```python
from build123d import *

# Parameters (mm, degrees)
F0_W     = 118.5
F0_H     = 123.5
F1_DEPTH = 1
F2_W     = 110
F2_H     = 115
F3_DEPTH = 25
F5_DEPTH = 1


with BuildPart() as f1:
    # F0 (on Top) → F1 (new body)
    with BuildSketch(Plane.XY):
        Rectangle(F0_W, F0_H)
    extrude(amount=F1_DEPTH)

    # F2 (on face) → F3 (cut)
    with BuildSketch(Plane.XY.offset(1)):
        Rectangle(F2_W, F2_H)
    extrude(amount=-F3_DEPTH, mode=Mode.SUBTRACT)

    # F4 (on Top) → F5 (join)
    with BuildSketch(Plane.XY):
        Polygon((2.5, 2.5), (2.5, 57.5), (-2.5, 57.5), (-2.5, 2.5), (-55, 2.5), (-55, -2.5), (-2.5, -2.5), (-2.5, -57.5), (2.5, -57.5), (2.5, -2.5), (55, -2.5), (55, 2.5), align=None)
    extrude(amount=F5_DEPTH)


solid = f1.part
```
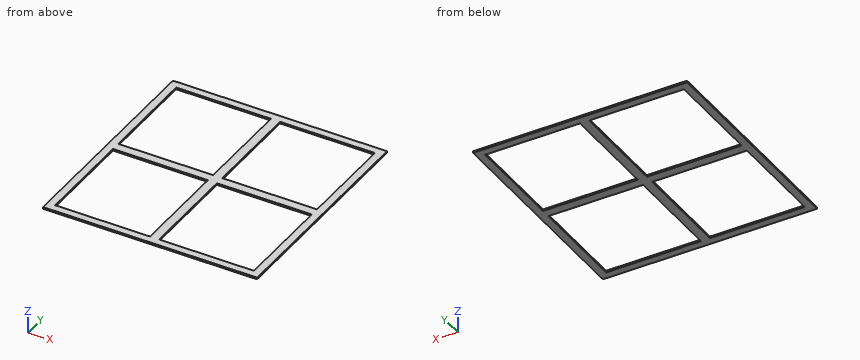
Check sheet for the modelled part. Datum: model origin and axes. Units: mm. Coordinates: 2 decimals unless noted, no trailing zeros. Loops run counter-clockwise (first coordinate to the right, second up) from the corner with the lowest first, then second, coordinate; pieces in that order, holes last.
1) Material ranges on probe 1 along X at (y, z) = (44.5, 0.15); probe 2 along Y at (x, z) = (-38, 0.9), recorded low to high.
2) Sectioned sample at B-B (x = -43.5). Record the boundary of the cut face in (y, z).
3) Sectioned sample at A-A (y = -23). Record the boundary of the cut face in (x, z), and give its area (3 significant figures).
4) Sectioned sample at C-C (z = 0.35). Record the boundary of the cut face in (x, y), and give its area (3 significant figures).
Check sheet entries:
1. probe 1: x = -59.25 to -55, -2.5 to 2.5, 55 to 59.25
1. probe 2: y = -61.75 to -57.5, -2.5 to 2.5, 57.5 to 61.75
2. outline: (-61.75, 0) - (-57.5, 0) - (-57.5, 1) - (-61.75, 1) - close; (-2.5, 0) - (2.5, 0) - (2.5, 1) - (-2.5, 1) - close; (57.5, 0) - (61.75, 0) - (61.75, 1) - (57.5, 1) - close
3. outline: (-59.25, 0) - (-55, 0) - (-55, 1) - (-59.25, 1) - close; (-2.5, 0) - (2.5, 0) - (2.5, 1) - (-2.5, 1) - close; (55, 0) - (59.25, 0) - (59.25, 1) - (55, 1) - close
3. area: 13.5 mm2
4. outline: (-59.25, -61.75) - (59.25, -61.75) - (59.25, 61.75) - (-59.25, 61.75) - close; hole (-55, -57.5) - (-2.5, -57.5) - (-2.5, -2.5) - (-55, -2.5) - close; hole (-55, 2.5) - (-2.5, 2.5) - (-2.5, 57.5) - (-55, 57.5) - close; hole (2.5, -57.5) - (55, -57.5) - (55, -2.5) - (2.5, -2.5) - close; hole (2.5, 2.5) - (55, 2.5) - (55, 57.5) - (2.5, 57.5) - close
4. area: 3,080 mm2
